Geometry check sheet. Reference: the model listing, model coordinates, mm. A direction names the side the tool comes from. Coordinates: 2 decimals unless noted, no trailing zeros. Write each loop counter-clockwise with the first axis right and the second up, starting at its lowest first coordinate (ties: lowest second). Pieces come first, ordered by that corner, then holes. Notation, with made-up numbers: (22.25, -29) -> (79.25, -29) arc R34 cw to (79.25, 8) -> close; hole circle Ø8 at (-0.75, -37.5). An arc over 180 degrees is marked (long way). One line per question, with ' | ' between items.
```python
from build123d import *

# Parameters (mm, degrees)
CROQUIS1_R              = 40
CROQUIS1_R_2            = 12.5
SALIENTE_EXTRUIR1_DEPTH = 50
CROQUIS2_R              = 2.5
CORTAR_EXTRUIR1_DEPTH   = 20
CROQUIS3_R              = 2.5
CORTAR_EXTRUIR2_DEPTH   = 20
CROQUIS4_R              = 2.5
CORTAR_EXTRUIR3_DEPTH   = 20
CROQUIS5_R              = 2
CORTAR_EXTRUIR4_DEPTH   = 20
CROQUIS6_R              = 2
CORTAR_EXTRUIR5_DEPTH   = 20
CROQUIS7_R              = 2
CORTAR_EXTRUIR6_DEPTH   = 20
REDONDEO1_R             = 20


with BuildPart() as part:
    # Croquis1 → Saliente-Extruir1 (new body)
    with BuildSketch(Plane.XY):
        Circle(CROQUIS1_R)
        Circle(CROQUIS1_R_2, mode=Mode.SUBTRACT)
    extrude(amount=SALIENTE_EXTRUIR1_DEPTH)

    # Croquis2 → Cortar-Extruir1 (cut)
    with BuildSketch(Plane(origin=(34.641016151, -20, 0), x_dir=(0, 0, -1), z_dir=(0.8660254037844364, -0.5000000000000041, 0))):
        with Locations(Location((-25, 0, 0), (0, 0, 90))):
            Circle(CROQUIS2_R)
    extrude(amount=-CORTAR_EXTRUIR1_DEPTH, mode=Mode.SUBTRACT)

    # Croquis3 → Cortar-Extruir2 (cut)
    with BuildSketch(Plane(origin=(0, 40, 0), x_dir=(1, 0, 0), z_dir=(0, 1, 0))):
        with Locations(Location((0, -25, 0), (0, 0, 270))):
            Circle(CROQUIS3_R)
    extrude(amount=-CORTAR_EXTRUIR2_DEPTH, mode=Mode.SUBTRACT)

    # Croquis4 → Cortar-Extruir3 (cut)
    with BuildSketch(Plane(origin=(-34.641016151, -20, 0), x_dir=(0, 0, -1), z_dir=(-0.8660254037844398, -0.499999999999998, 0))):
        with Locations(Location((-25, 0, 0), (0, 0, 90))):
            Circle(CROQUIS4_R)
    extrude(amount=-CORTAR_EXTRUIR3_DEPTH, mode=Mode.SUBTRACT)

    # Croquis5 → Cortar-Extruir4 (cut)
    with BuildSketch(Plane(origin=(-34.641016151, -20, 0), x_dir=(0, 0, -1), z_dir=(-0.8660254037844398, -0.499999999999998, 0))):
        with Locations(Location((-7.32233047, 17.67766953, 0), (0, 0, 90))):
            Circle(CROQUIS5_R)
    extrude(amount=-CORTAR_EXTRUIR4_DEPTH, mode=Mode.SUBTRACT)

    # Croquis6 → Cortar-Extruir5 (cut)
    with BuildSketch(Plane(origin=(34.641016151, -20, 0), x_dir=(0, 0, -1), z_dir=(0.8660254037844364, -0.5000000000000041, 0))):
        with Locations(Location((-7.32233047, 17.67766953, 0), (0, 0, 90))):
            Circle(CROQUIS6_R)
    extrude(amount=-CORTAR_EXTRUIR5_DEPTH, mode=Mode.SUBTRACT)

    # Croquis7 → Cortar-Extruir6 (cut)
    with BuildSketch(Plane(origin=(0, 40, 0), x_dir=(1, 0, 0), z_dir=(0, 1, 0))):
        with Locations(Location((-17.67766953, -7.32233047, 0), (0, 0, 270))):
            Circle(CROQUIS7_R)
    extrude(amount=-CORTAR_EXTRUIR6_DEPTH, mode=Mode.SUBTRACT)

    # Croquis8 → Revolución1 (revolve)
    with BuildSketch(Plane(origin=(0, 0, 0), x_dir=(1, 0, 0), z_dir=(0, 1, 0))):
        with BuildLine():
            Line((0, 0), (40, 0))
            Line((40, 0), (1.723076923, 66.984615385))
            ThreePointArc((1.723076923, 66.984615385), (0.996101755, 67.716462301), (0, 67.984555753))
            Line((0, 67.984555753), (0, 64.015444247))
            Line((0, 64.015444247), (0, 0))
        make_face()
    revolve(axis=Axis((0, 0, 0), (0, 0, -1)))

    # Redondeo1
    redondeo1_edges = [part.edges().sort_by_distance(p)[0] for p in [
        (-40, 0, 0),
    ]]
    fillet(redondeo1_edges, radius=REDONDEO1_R)


solid = part.part
```
(1) Cross-section at D-D (z = -32). Record the cut outline in (x, y), plus the area to 3 significant figures.
Answers below:
outline: circle Ø43.43 at (0, 0) | area: 1,480 mm²
(2) Cross-section at B-B (z = -58.5). Record the cut outline in (x, y).
Answers below:
outline: circle Ø13.14 at (0, 0)
(3) Cross-section at A-A (z = 25). Record the cut outline in (x, y), plus the area to 3 significant figures.
Answers below:
outline: (-35.82, -17.8) -> (-18.57, -7.83) -> (-16.07, -12.17) -> (-33.32, -22.13) arc R40 ccw to (33.32, -22.13) -> (16.07, -12.17) -> (18.57, -7.83) -> (35.82, -17.8) arc R40 ccw to (2.5, 39.92) -> (2.5, 20) -> (-2.5, 20) -> (-2.5, 39.92) arc R40 ccw to start; hole circle Ø25 at (0, 0) | area: 4,240 mm²
(4) Tool access check on faces 1 (the face through (26.15, 5.29, 7.35)), 2 (the face through (-3.32, 14.97, -43.17)), 3 (the face through (11.923, 3.755, 24.65)), 4 (the face through (38.153, 12.015, 27.334)), 5 (the face through (-15.695, 28.517, 7.062)). Record the directions out of +Z, -Z, +X, -X, +Y, -Y that give a thin tool (end or side, any length) a straight path to the whole face; none if there is none.
Answers below:
face 1: none | face 2: -Z | face 3: +Z | face 4: +Z, -Z | face 5: +Y
(5) Depth check by flat-ended pin: P1, Ø2, axis at x = 18.5, z = -16.5, coming from the +Y side; P2, Ø5, axis at y = -30.5, z = -15.5, coming from the -X side; P3, Ø20, axis at x = 5.5, y = -1.5, coming from the +Z side; P4, Ø4.5, axis at x = -17.68, z = 7.32, coming from the -Y side. Enter the tip coordinate at first touch or a pass-through.
Answers below:
P1: stops at y = 25.36 | P2: stops at x = -14.57 | P3: stops at z = 50 | P4: stops at y = -36.9
(6) Draft check along Y on faces 6 (the face through (0, 20, 25)), 7 (the face through (-26.26, -14.79, 27.48)), 8 (the face through (-9, 9, 50)). Enter one of: pulls with the +Y half, pulls with the -Y half, needs draft (parallel to the pull), parting line crosses it, or undercut.
Answers below:
face 6: pulls with the +Y half | face 7: undercut | face 8: needs draft
(7) Cross-section at C-C (y = 33.5). Count the separate pieces of the cut face and the enclosed holes in it, plus the area to 3 significant figures.
Answers below:
separate pieces: 1 | enclosed holes: 2 | area: 2,470 mm²
(8) Material ranges on line 1 (Y direction, x = 0, z = 15.5); line 2 (Y direction, x = 2, z = 18), recorded low to high.
Answers below:
line 1: y = -40 to -12.5, 12.5 to 40 | line 2: y = -39.95 to -12.34, 12.34 to 39.95
